Can you work these out from the drawing? Everything is in mm from the part's minimum corner. Coordinates: 2 decimals unless noted, no trailing zeros. Order: outer loops, then holes, each group sorted by start corner. A loop starts at its lowest first (then second) coordinate and runs counter-clockwise, first axis right, second up. Notation, with made-up numbers: M 67,87 L 104,87 A14 cw 104,114 Z; hole C 32,78 d5. An arc over 180 degrees is marked long. One line per question, with ' | ' between items. Start each with the question number.
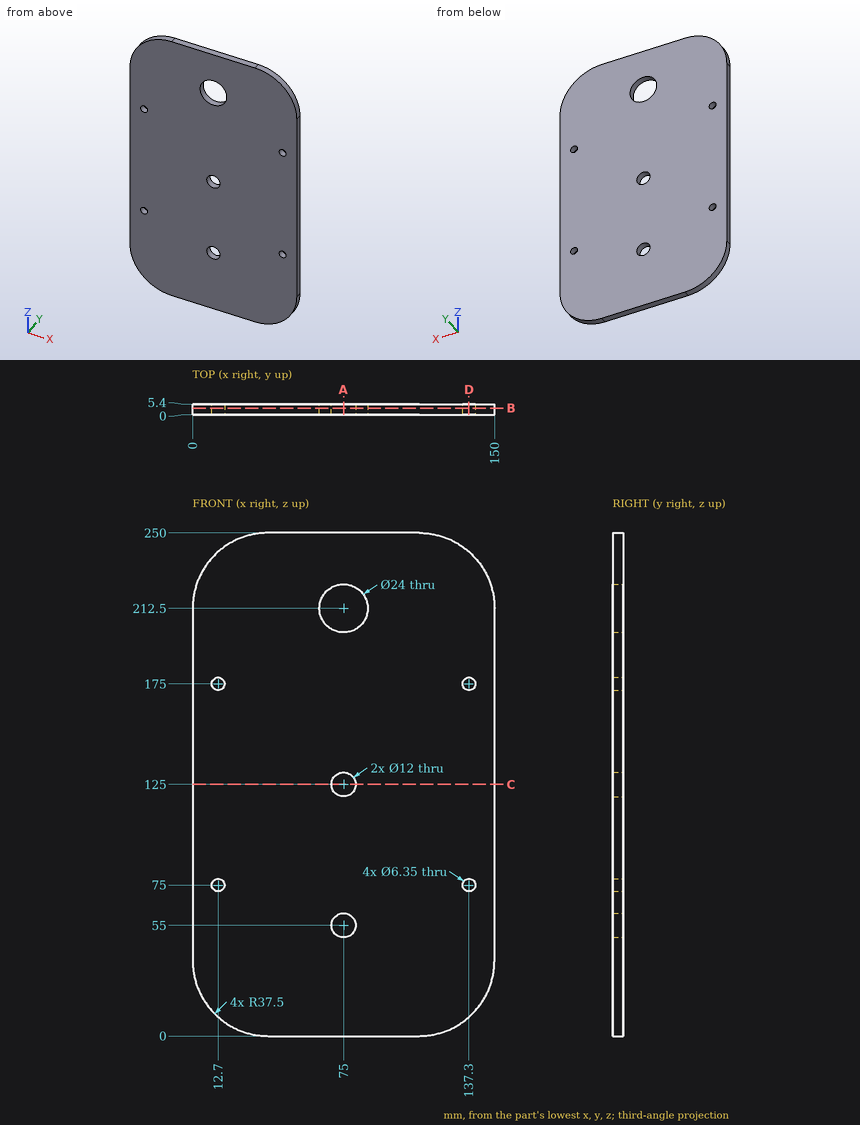
(1) Imagine slicing it at A-A, the plane x = 75. Write out the boundary of the cut face in (y, z), plus the area to 3 significant figures.
(2) Imagine slicing it at C-C, the plane z = 125. Write out the boundary of the cut face in (x, y).
(3) Imagine slicing it at D-D, the plane x = 137.3. Write out the boundary of the cut face in (y, z) (3 decimals).
(4) If I drill on line 1 along X through (y, z) = (1.65, 175) (3 decimals); line 2 along X through (y, z) = (4.75, 175.5); line 3 along Z through (x, y) = (137.3, 2.1) (3 decimals), over which ranges is the centre line in solid material (lowest first)? Write a range as from..to.
(5) Imagine slicing it at B-B, the plane y = 3.3. Write out the boundary of the cut face in (x, z) (3 decimals), plus the area to 3 significant figures.
Answers:
1) outline: M 0,0 L 5.4,0 L 5.4,49 L 0,49 Z; M 0,61 L 5.4,61 L 5.4,119 L 0,119 Z; M 0,131 L 5.4,131 L 5.4,200.5 L 0,200.5 Z; M 0,224.5 L 5.4,224.5 L 5.4,250 L 0,250 Z | area: 1,090 mm²
2) outline: M 0,0 L 69,0 L 69,5.4 L 0,5.4 Z; M 81,0 L 150,0 L 150,5.4 L 81,5.4 Z
3) outline: M 0,9.372 L 5.4,9.372 L 5.4,71.825 L 0,71.825 Z; M 0,78.175 L 5.4,78.175 L 5.4,171.825 L 0,171.825 Z; M 0,178.175 L 5.4,178.175 L 5.4,240.628 L 0,240.628 Z
4) line 1: 0..9.525, 15.875..134.125, 140.475..150 | line 2: 0..9.56, 15.84..134.16, 140.44..150 | line 3: 9.372..71.825, 78.175..171.825, 178.175..240.628
5) outline: M 0,37.5 A37.5 ccw 37.5,0 L 112.5,0 A37.5 ccw 150,37.5 L 150,212.5 A37.5 ccw 112.5,250 L 37.5,250 A37.5 ccw 0,212.5 Z; hole C 12.7,75 d6.35; hole C 12.7,175 d6.35; hole C 75,212.5 d24; hole C 75,55 d12; hole C 75,125 d12; hole C 137.3,75 d6.35; hole C 137.3,175 d6.35 | area: 35,500 mm²
